```python
from build123d import *

# Parameters (mm, degrees)
CUT_EXTRUDE1_DEPTH      = 257.457873087
CUT_EXTRUDE1_DEPTH_BACK = 257.457873087
SKETCH5_R               = 6.35
CUT_EXTRUDE4_DEPTH      = 257.457873098
SKETCH6_R               = 16.711436386
SKETCH6_R_2             = 17.485757022
CUT_EXTRUDE5_DEPTH      = 257.83197321
SKETCH7_W               = 38.686396819
SKETCH7_H               = 81.826205817
CUT_EXTRUDE6_DEPTH      = 257.457873098
CUT_EXTRUDE7_DEPTH      = 257.457873098
CUT_EXTRUDE7_DEPTH_BACK = 257.457873098
CUT_EXTRUDE8_START      = -3.381369738
CUT_EXTRUDE8_DEPTH      = 30.084768361


# Read off the part's stored shape, not the designer's step: Cut-Extrude8
with BuildPart() as part:
    # Sweep2: sweep along a path in Sketch1
    with BuildLine(Plane.XY) as sweep2_path:
        CenterArc((0, 0), 139.7, 0, 360)
    # Sketch2 → Sweep2 (sweep)
    with BuildSketch(Plane(origin=(0, 0, 0), x_dir=(0, 0, -1), z_dir=(1, 0, 0))):
        Polygon((0.081951645, 85.453687679), (0, 143.147726507), (-26.703398523, 180.357380187), (-23.40398043, 180.357380187), (3.381369738, 143.033531592), (3.381369738, 85.453687679), align=None)
    sweep(path=sweep2_path.line)

    # Sketch3 → Cut-Extrude1 (cut, two sides: drawn at the far end of the back side and taken through both)
    with BuildSketch(Plane.XY.offset(-CUT_EXTRUDE1_DEPTH_BACK)):
        Polygon((821.723604832, 900.839301856), (152.923564845, 137.799256234), (60.497234444, 32.34921564), (-41.171728997, -70.159987168), (-55.875917924, -70.159987168), (-55.875917924, -126.035905092), (-167.627753772, -126.035905092), (-167.627753772, -181.911823016), (-167.627753772, -1196.566249267), (1667.740204928, -2062.313830848), (2657.091563532, 35.091720274), align=None)
    extrude(amount=CUT_EXTRUDE1_DEPTH + CUT_EXTRUDE1_DEPTH_BACK, mode=Mode.SUBTRACT)

    # Sketch5 → Cut-Extrude4 (cut, through all)
    with BuildSketch(Plane.XY):
        with Locations((-76.174636448, 78.185490602)):
            Circle(SKETCH5_R)
        with Locations((-76.260331952, -75.414325116)):
            Circle(SKETCH5_R)
    extrude(amount=-CUT_EXTRUDE4_DEPTH, mode=Mode.SUBTRACT)

    # Sketch6 → Cut-Extrude5 (cut, through all)
    with BuildSketch(Plane(origin=(0, 0, -3.381369738), x_dir=(-1, 0, 0), z_dir=(0, 0, -1))):
        with Locations((0, 109.236739893)):
            Circle(SKETCH6_R)
        with Locations((112.112202079, 0)):
            Circle(SKETCH6_R_2)
    extrude(amount=-CUT_EXTRUDE5_DEPTH, mode=Mode.SUBTRACT)

    # Sketch7 → Cut-Extrude6 (cut, through all)
    with BuildSketch(Plane.XY):
        with Locations((-36.532719515, -85.122802183)):
            Rectangle(SKETCH7_W, SKETCH7_H)
    extrude(amount=-CUT_EXTRUDE6_DEPTH, mode=Mode.SUBTRACT)

    # Sketch8 → Cut-Extrude7 (cut, two sides: drawn at the far end of the back side and taken through both)
    with BuildSketch(Plane.XY.offset(-CUT_EXTRUDE7_DEPTH_BACK)):
        with BuildLine():
            Line((517.613905497, -613.797286977), (111.177648296, 90.170960534))
            Line((111.177648296, 90.170960534), (95.308152083, 117.657734266))
            ThreePointArc((95.308152083, 117.657734266), (92.009440132, 125.621529396), (90.884310916, 134.167734266))
            Line((90.884310916, 134.167734266), (90.884310916, 169.901611192))
            Line((90.884310916, 169.901611192), (90.884310916, 982.774125595))
            Line((90.884310916, 982.774125595), (1661.496369245, 1402.565336698))
            Line((1661.496369245, 1402.565336698), (2088.225963826, -194.006075874))
            Line((2088.225963826, -194.006075874), (517.613905497, -613.797286977))
        make_face()
    extrude(amount=CUT_EXTRUDE7_DEPTH + CUT_EXTRUDE7_DEPTH_BACK, mode=Mode.SUBTRACT)

    # Cut-Extrude8 outline → Cut-Extrude8 (cut)
    with BuildSketch(Plane.XY.offset(CUT_EXTRUDE8_START)):
        with BuildLine():
            Line((90.884310916, 155.784551921), (33.711604752, 78.522993084))
            ThreePointArc((33.711604752, 78.522993084), (55.441528266, 65.02745329), (72.203661887, 45.705185132))
            Line((72.203661887, 45.705185132), (111.177648296, 90.170960534))
            Line((111.177648296, 90.170960534), (95.308152083, 117.657734266))
            ThreePointArc((95.308152083, 117.657734266), (92.009440132, 125.621529397), (90.884310916, 134.167734266))
            Line((90.884310916, 134.167734266), (90.884310916, 155.784551921))
        make_face()
    extrude(amount=CUT_EXTRUDE8_DEPTH, mode=Mode.SUBTRACT)


solid = part.part
```
Verification items for the finished model (mm, model axes). Coordinates: 2 decimals unless noted, no trailing zeros. Loops run counter-clockwise (first coordinate to the right, second up) from the corner with the lowest first, then second, coordinate; pieces in that order, holes last. Notation, with made-up numbers: (53.5, 16) - (85.5, 16) arc R12 cw to (85.5, 21) - close; hole circle Ø7 at (0.5, -19.75). An arc over 180 degrees is marked (long way). Answer as a JSON object with one key per item and string values.
(1) Scan lines: line 1 along Z through (x, y) = (-108.5, 64.5); line 2 along Y through (x, z) = (0, -2); line 3 along Z through (x, y) = (-94, -51). Record each from-to range of solid material in increasing order.
Response:
{"line 1": "z = -3.38 to -0.02", "line 2": "y = 85.45 to 92.53, 125.95 to 144.96", "line 3": "z = -3.38 to -0.05"}
(2) Cross-section at A-A, the plane z = 13. Record the boundary of the cut face in (x, y).
Response:
{"outline": "(-107.82, -126.04) - (-100.6, -126.04) arc R161.26 cw to (79.45, 140.33) - (82.2, 144.06) arc R165.86 ccw to start"}
(3) Mould release check, pull along X, two halves, no side actions. Record for faces 1 (the conical face through (-125.238, 73.807, -1.706)), 2 (the conical face through (-124.83, 73.69, 1.3)), 3 (the flat face through (-92, -126.036, 9)): pulls with the +X half, pulls with the -X half, needs draft (parallel to the pull), parting line crosses it, or undercut.
Response:
{"face 1": "parting line crosses it", "face 2": "undercut", "face 3": "needs draft"}
(4) Go/stop test with flat-tipped pins: pin 1 Ø3 at (x, z) = (46, 9.5) entering from -Y; pin 2 Ø2.5 at (y, z) = (-99, -2) entering from +X; pin 3 Ø11.5 at (x, y) = (-76.26, -75.41) entering from -Z; pin 4 Ø2 at (y, z) = (-19, 20) entering from +X. Record where each tip stops, or that it passes through.
Response:
{"pin 1": "stops at y = 147.23", "pin 2": "stops at x = -55.88", "pin 3": "passes through", "pin 4": "stops at x = -168.55"}
